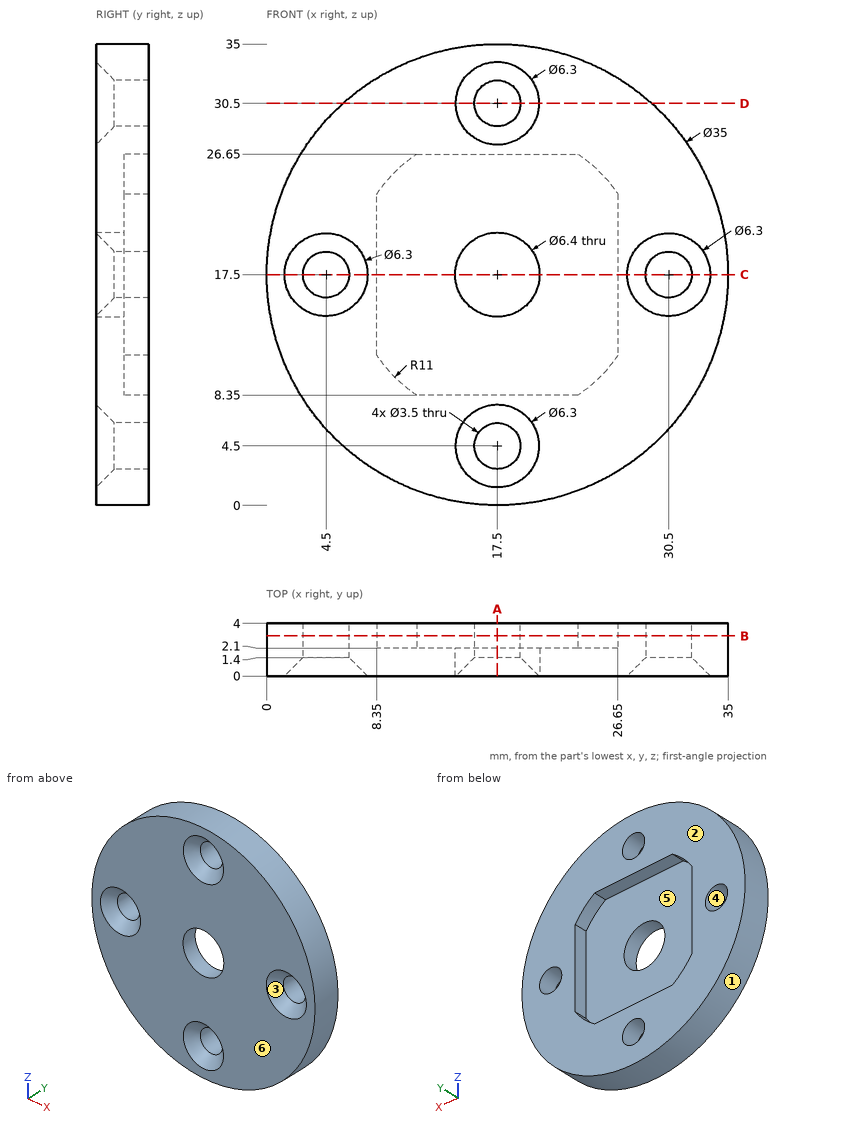
Input: dimensioned drawing with shaded views. Units: mm. Origin: part minimum x, y, z. A direction names the side the tool comes from. Coordinates: 2 decimals unless noted, no trailing zeros. Order: outer loops, then holes, each group sorted by start corner. A loop starts at its lowest first (then second) coordinate and runs counter-clockwise, first axis right, second up. Notation, with made-up numbers: (80.25, -15) -> (87.25, -15) arc R12 ccw to (87.25, 3) -> close; hole circle Ø3 at (43, 56). An arc over 180 degrees is marked (long way). Use CSV: the item, a comma, the result in double quotes.
1) Line query: line 1 (Z direction, x = 17.5, y = 2.4); line 2 (X direction, y = 2, z = 17.5). Output: solid intervals per line, ascending.
Findings:
line 1,"z = 0 to 2.75, 6.25 to 8.35, 26.65 to 28.75, 32.25 to 35"
line 2,"x = 0 to 2.75, 6.25 to 14.3, 20.7 to 28.75, 32.25 to 35"
2) Access query for the marked faces 5 and 6. Directions: +Z, -Z, +X, -X, +Y, -Y. A direction counts if a zero-diameter tool reaches every point of the face in a straight line with its end or side. Return the directions, or none.
Findings:
face 5,"+Y"
face 6,"+Z, -Z, +X, -X, -Y"
3) Pin query (flat end, axial travel): pin 1 Ø4.5 at (x, z) = (17.5, 4.5) entering from -Y; pin 2 Ø1 at (x, y) = (5, 1) entering from +Z; pin 3 Ø2 at (y, z) = (1.5, 14.5) entering from +X. Return the tip coordinate at first contact, or that it passes through.
Findings:
pin 1,"stops at y = 0.9"
pin 2,"stops at z = 30.24"
pin 3,"stops at x = 34.89"
4) Section C-C on z = 17.5. Output: boundary loops of the cut face in (x, y), then the cut area to 3 significant figures.
Findings:
outline,"(0, 0) -> (1.35, 0) -> (2.75, 1.4) -> (2.75, 4) -> (0, 4) -> close; (6.25, 1.4) -> (7.65, 0) -> (14.3, 0) -> (14.3, 2.1) -> (8.35, 2.1) -> (8.35, 4) -> (6.25, 4) -> close; (20.7, 0) -> (27.35, 0) -> (28.75, 1.4) -> (28.75, 4) -> (26.65, 4) -> (26.65, 2.1) -> (20.7, 2.1) -> close; (32.25, 1.4) -> (33.65, 0) -> (35, 0) -> (35, 4) -> (32.25, 4) -> close"
area,"59.9 mm^2"
5) Section B-B on y = 3.05. Output: boundary loops of the cut face in (x, z), then the cut area to 3 significant figures.
Findings:
outline,"circle Ø35 at (17.5, 17.5); hole circle Ø3.5 at (4.5, 17.5); hole (8.35, 11.39) arc R11 ccw to (11.39, 8.35) -> (23.61, 8.35) arc R11 ccw to (26.65, 11.39) -> (26.65, 23.61) arc R11 ccw to (23.61, 26.65) -> (11.39, 26.65) arc R11 ccw to (8.35, 23.61) -> close; hole circle Ø3.5 at (17.5, 4.5); hole circle Ø3.5 at (17.5, 30.5); hole circle Ø3.5 at (30.5, 17.5)"
area,"605 mm^2"
6) Section D-D on z = 30.5. Output: boundary loops of the cut face in (x, y), then the cut area to 3 significant figures.
Findings:
outline,"(5.78, 0) -> (14.35, 0) -> (15.75, 1.4) -> (15.75, 4) -> (5.78, 4) -> close; (19.25, 1.4) -> (20.65, 0) -> (29.22, 0) -> (29.22, 4) -> (19.25, 4) -> close"
area,"77.8 mm^2"
7) Mould query, pull axis X, two halves, no side actions, for the marked faces 1, 2, 3 and 4. Classes: +X half, -X half, draft (parallel to the pull), parting line (faces both ways), or undercut.
Findings:
face 1,"parting line"
face 2,"draft"
face 3,"undercut"
face 4,"undercut"
8) Section A-A on x = 17.5. Output: boundary loops of the cut face in (y, z), then the cut area to 3 significant figures.
Findings:
outline,"(0, 0) -> (4, 0) -> (4, 2.75) -> (1.4, 2.75) -> (0, 1.35) -> close; (0, 7.65) -> (1.4, 6.25) -> (4, 6.25) -> (4, 8.35) -> (2.1, 8.35) -> (2.1, 14.3) -> (0, 14.3) -> close; (0, 20.7) -> (2.1, 20.7) -> (2.1, 26.65) -> (4, 26.65) -> (4, 28.75) -> (1.4, 28.75) -> (0, 27.35) -> close; (0, 33.65) -> (1.4, 32.25) -> (4, 32.25) -> (4, 35) -> (0, 35) -> close"
area,"59.9 mm^2"
